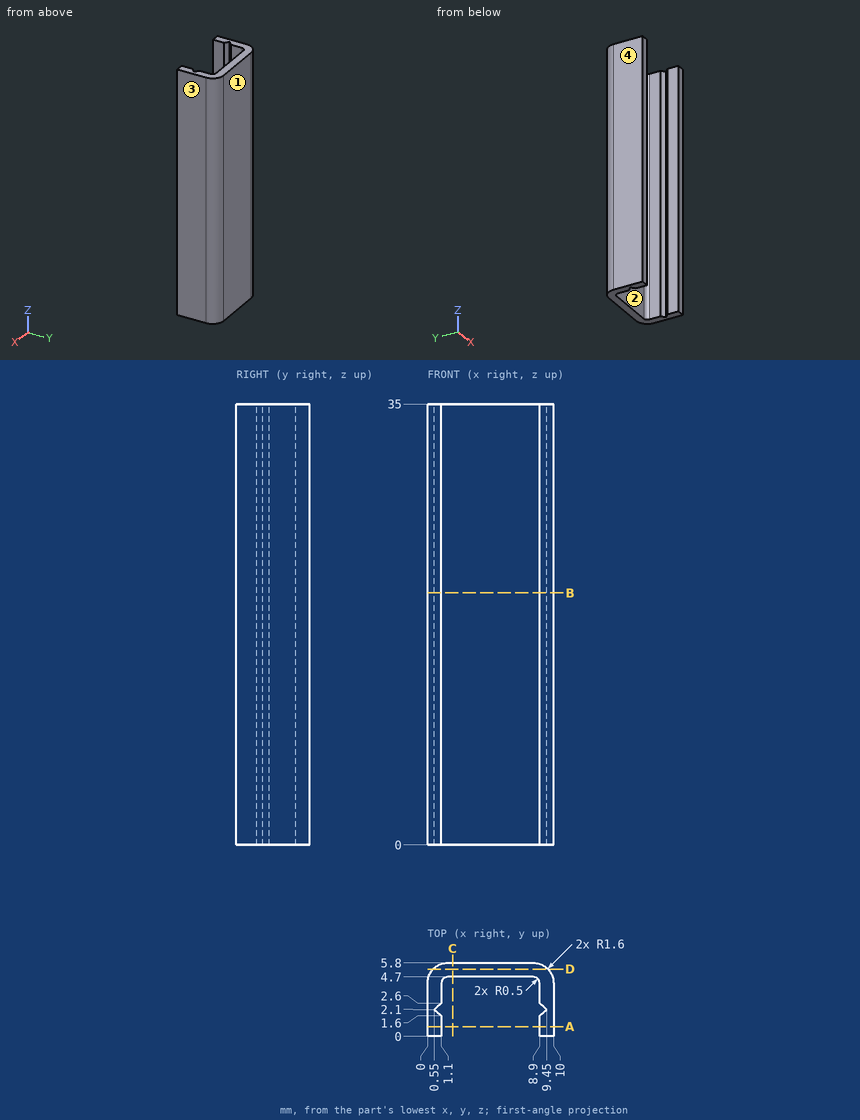
Check sheet for the drawn part. Datum: minimum x, y, z corner. Units: mm. Coordinates: 2 decimals unless noted, no trailing zeros. Order: outer loops, then holes, each group sorted by start corner. A loop starts at its lowest first (then second) coordinate and runs counter-clockwise, first axis right, second up. Notation, with made-up numbers: M 45.25,-35.5 L 56.25,-35.5 A28 ccw 56.25,-15.5 Z; hole C -8,66.5 d5. An arc over 180 degrees is marked long. One line per item, written item: value. Start each with the question number.
Item 1: Gauge pin test, flat ends, axial feed: pin 1 (3 mm diameter, centred on y = 1.5, z = 24.5, fed in from -X); pin 2 (1.5 mm diameter, centred on x = 2.5, z = 9.5, fed in from -Y). Record the tip position at first contact, or that the pin passes through.
Item 2: Mould release check, pull along X, two halves, no side actions. Record for the marked faces 1, 2, 3 and 4: released by +X, released by -X, zero draft, split by the parting line, or undercut.
Item 3: Sectioned sample at B-B (z = 20). Enter the section's corners in (x, y), then the cut area to 3 significant figures.
Item 4: Sectioned sample at C-C (x = 2). Enter the section's corners in (y, z), then the cut area to 3 significant figures.
Item 5: Sectioned sample at A-A (y = 0.75). Enter the section's corners in (x, z), then the cut area to 3 significant figures.
Item 6: Scan lines: probe 1 along X at (y, z) = (3.4, 23); probe 2 along Y at (x, z) = (7.75, 28); probe 3 along X at (y, z) = (2.2, 33). Record each from-to range of solid material in increasing order.
Item 7: Sectioned sample at D-D (y = 5.3). Enter the section's corners in (x, z), then the cut area to 3 significant figures.
Conclusion:
1. pin 1: stops at x = 0
1. pin 2: stops at y = 4.7
2. face 1: zero draft
2. face 2: undercut
2. face 3: released by +X
2. face 4: released by -X
3. outline: M 0,0 L 1.1,0 L 1.1,1.6 L 0.55,2.1 L 1.1,2.6 L 1.1,4.2 A0.5 cw 1.6,4.7 L 8.4,4.7 A0.5 cw 8.9,4.2 L 8.9,2.6 L 9.45,2.1 L 8.9,1.6 L 8.9,0 L 10,0 L 10,4.2 A1.6 ccw 8.4,5.8 L 1.6,5.8 A1.6 ccw 0,4.2 Z
3. area: 19.8 mm^2
4. outline: M 4.7,0 L 5.8,0 L 5.8,35 L 4.7,35 Z
4. area: 38.5 mm^2
5. outline: M 0,0 L 1.1,0 L 1.1,35 L 0,35 Z; M 8.9,0 L 10,0 L 10,35 L 8.9,35 Z
5. area: 77.0 mm^2
6. probe 1: x = 0 to 1.1, 8.9 to 10
6. probe 2: y = 4.7 to 5.8
6. probe 3: x = 0 to 0.66, 9.34 to 10
7. outline: M 0.44,0 L 9.56,0 L 9.56,35 L 0.44,35 Z
7. area: 319 mm^2
